from build123d import *

# Parameters (mm, degrees)
SKETCH1_W           = 31.75
SKETCH1_H           = 7.75
BOSS_EXTRUDE1_DEPTH = 9.6
SKETCH2_R           = 2.45
BOSS_EXTRUDE2_DEPTH = 1.8
SHELL1_T            = -1.5


with BuildPart() as part:
    # Sketch1 → Boss-Extrude1 (new body)
    with BuildSketch(Plane(origin=(0, 0, 0), x_dir=(1, 0, 0), z_dir=(0, 1, 0))):
        Rectangle(SKETCH1_W, SKETCH1_H)
    extrude(amount=-BOSS_EXTRUDE1_DEPTH)

    # Sketch2 → Boss-Extrude2 (add)
    with BuildSketch(Plane(origin=(0, 0, 0), x_dir=(1, 0, 0), z_dir=(0, 1, 0))):
        with Locations(Location((-11.94, 0, 0), (0, 0, 270))):
            Circle(SKETCH2_R)
        with Locations(Location((-3.98, 0, 0), (0, 0, 270))):
            Circle(SKETCH2_R)
        with Locations(Location((3.98, 0, 0), (0, 0, 270))):
            Circle(SKETCH2_R)
        with Locations(Location((11.94, 0, 0), (0, 0, 270))):
            Circle(SKETCH2_R)
    extrude(amount=BOSS_EXTRUDE2_DEPTH)

    # Shell1
    shell1_openings = [part.faces().sort_by_distance(p)[0] for p in [
        (0, -9.6, 0),
    ]]
    offset(amount=SHELL1_T, openings=shell1_openings, kind=Kind.INTERSECTION)


solid = part.part
Work out the finished part from the listing and answer in its coordinate system (mm). A direction names the side the tool comes from. Round coordinates to 2 decimals unless told otherwise and drop trailing zeros. Loops run counter-clockwise (first coordinate to the right, second up) from the corner with the lowest first, then second, coordinate; pieces in that order, holes last. Notation, with made-up numbers: (30.5, 88.25) - (49.5, 88.25) arc R12 cw to (49.5, 102.25) - close; hole circle Ø4 at (56, 6.25). An arc over 180 degrees is marked (long way). Use one line per item in the form item = value. Start each with the question number.
(1) Find section D-D on x = -7. Determine the outline of the cut face in (y, z) (3 decimals).
(2) Find section A-A on y = -7.25. Determine the outline of the cut face in (x, z) (3 decimals), and give its area (4 significant figures).
(3) Consider line 1 (X direction, y = -0.9, z = 0) (3 decimals); line 2 (Z direction, x = -3.98, y = -0.2) (3 decimals); line 3 (Z direction, x = 14, y = -3.25) (3 decimals). Determine where each line is inside the solid, lowest interval first.
(4) Flat-ended cylindrical pins translate along their axes: P1, Ø2.5, axis at x = -11.94, z = 0, coming from the -Y side; P2, Ø0.6, axis at x = -4.5, z = 0, coming from the -Y side. Find the tip coordinate at first contact, or state that the pin passes through.
(5) Determine the mould class of faces 4 (the face through (15.875, -5, 0)), 5 (the face through (0, -5, 3.875)), 6 (the face through (0, -5, 2.375)) for opening direction X: +X half, -X half, draft (parallel to the pull), parting line (faces both ways), or undercut.
(6) Which of the six approach directions +Z, -Z, +X, -X, +Y, -Y give full straight-line access (tool end or side, diameter ignored) to faces 1 (the face through (-12, 0.3, 0)), 2 (the face through (-4, 1.8, 0)), 3 (the face through (-1.914, 0.887, 1.317))?
(7) Find section B-B on x = 11.94. Determine the outline of the cut face in (y, z) (3 decimals), and give its area (3 significant figures).
(8) Find section C-C on z = 1.5. Determine the outline of the cut face in (x, y) (3 decimals), and give its area (3 significant figures).
Answer list:
q1.outline = (-9.6, -3.875) - (0, -3.875) - (0, 3.875) - (-9.6, 3.875) - (-9.6, 2.375) - (-1.5, 2.375) - (-1.5, -2.375) - (-9.6, -2.375) - close
q2.outline = (-15.875, -3.875) - (15.875, -3.875) - (15.875, 3.875) - (-15.875, 3.875) - close; hole (-14.375, -2.375) - (14.375, -2.375) - (14.375, 2.375) - (-14.375, 2.375) - close
q2.area = 109.5 mm^2
q3.line_1 = -15.875 to -12.89, -10.99 to -4.93, -3.03 to 3.03, 4.93 to 10.99, 12.89 to 15.875
q3.line_2 = -3.875 to -0.95, 0.95 to 3.875
q3.line_3 = -3.875 to -2.375, 2.375 to 3.875
q4.P1 = -1.5
q4.P2 = 0.3
q5.face_4 = +X half
q5.face_5 = draft
q5.face_6 = undercut
q6.face_1 = -Y
q6.face_2 = +Z, -Z, +X, -X, +Y
q6.face_3 = +Y
q7.outline = (-9.6, -3.875) - (0, -3.875) - (0, -2.45) - (1.8, -2.45) - (1.8, 2.45) - (0, 2.45) - (0, 3.875) - (-9.6, 3.875) - (-9.6, 2.375) - (-1.5, 2.375) - (-1.5, 0.95) - (0.3, 0.95) - (0.3, -0.95) - (-1.5, -0.95) - (-1.5, -2.375) - (-9.6, -2.375) - close
q7.area = 41.3 mm^2
q8.outline = (-15.875, -9.6) - (-14.375, -9.6) - (-14.375, -1.5) - (14.375, -1.5) - (14.375, -9.6) - (15.875, -9.6) - (15.875, 0) - (13.877, 0) - (13.877, 1.8) - (10.003, 1.8) - (10.003, 0) - (5.917, 0) - (5.917, 1.8) - (2.043, 1.8) - (2.043, 0) - (-2.043, 0) - (-2.043, 1.8) - (-5.917, 1.8) - (-5.917, 0) - (-10.003, 0) - (-10.003, 1.8) - (-13.877, 1.8) - (-13.877, 0) - (-15.875, 0) - close
q8.area = 99.8 mm^2
